```python
from build123d import *

# Parameters (mm, degrees)
F1_DEPTH  = 75
F2_W      = 55
F2_H      = 95
F3_DEPTH  = 3.001
F5_DEPTH  = 55
F7_DEPTH  = 3
F9_DEPTH  = 3
F10_R     = 2
F12_DEPTH = 3
F13_W     = 4
F13_H     = 3.0462798357
F14_DEPTH = 1


with BuildPart() as f1:
    # F0 (on Front) → F1 (new body)
    with BuildSketch(Plane.XZ):
        with BuildLine():
            Line((-3, 0), (0, 0))
            Line((0, 0), (0, 146.328642619))
            ThreePointArc((0, 146.328642619), (1.7690799336, 150.0361338491), (5.6451438845, 151.3967452123))
            Line((5.6451438845, 151.3967452123), (79.5057253604, 138.3731318873))
            Line((79.5057253604, 138.3731318873), (79.5057253604, 141.4194117229))
            Line((79.5057253604, 141.4194117229), (6.010801042, 154.3785498254))
            ThreePointArc((6.010801042, 154.3785498254), (-0.193413929, 152.3056303595), (-3, 146.396962731))
            Line((-3, 146.396962731), (-3, 146.1928579517))
            Line((-3, 146.1928579517), (-3, 0))
        make_face()
    extrude(amount=-F1_DEPTH)

    # F2 (on face) → F3 (cut, through all)
    with BuildSketch(Plane.YZ):
        with Locations((37.5, 47.5)):
            Rectangle(F2_W, F2_H)
    extrude(amount=-F3_DEPTH, mode=Mode.SUBTRACT)

    # F4 (on face) → F5 (join)
    with BuildSketch(Plane.XZ.offset(-65)):
        Polygon((0, 95), (-3, 95), (32.2094485164, 0), (47.2094485164, 0), (47.2094485164, 3), (34.2969885133, 3), align=None)
    extrude(amount=F5_DEPTH)

    # F6 (on face) → F7 (cut)
    with BuildSketch(Plane(origin=(0, 0, 0), x_dir=(1, 0, 0), z_dir=(0, 0, -1))):
        with BuildLine():
            ThreePointArc((42.2094485164, -37.5), (41.4772154693, -35.732233047), (39.7094485164, -35))
            Line((39.7094485164, -35), (39.7094485164, -40))
            ThreePointArc((39.7094485164, -40), (41.4772154693, -39.267766953), (42.2094485164, -37.5))
        make_face()
        with BuildLine():
            Line((39.7094485164, -40), (39.7094485164, -35))
            ThreePointArc((39.7094485164, -35), (37.2094485164, -37.5), (39.7094485164, -40))
        make_face()
    extrude(amount=-F7_DEPTH, mode=Mode.SUBTRACT)

    # F8 (on face) → F9 (cut, through all)
    with BuildSketch(Plane.YZ):
        with BuildLine():
            Line((7, 6), (7, 12))
            ThreePointArc((7, 12), (5, 14), (3, 12))
            Line((3, 12), (3, 6))
            ThreePointArc((3, 6), (5, 4), (7, 6))
        make_face()
        with BuildLine():
            ThreePointArc((72, 12), (70, 14), (68, 12))
            Line((68, 12), (68, 6))
            ThreePointArc((68, 6), (70, 4), (72, 6))
            Line((72, 6), (72, 12))
        make_face()
    extrude(amount=-F9_DEPTH, mode=Mode.SUBTRACT)

    # F10
    f10_edges = [f1.edges().sort_by_distance(p)[0] for p in [
        (32.209449, 37.5, 0),
        (34.296989, 37.5, 3),
    ]]
    fillet(f10_edges, radius=F10_R)

    # F11 (on face) → F12 (cut, through all)
    with BuildSketch(Plane(origin=(26.5815346978, 0, 150.7513744689), x_dir=(0.984807753, 0, -0.1736481777), z_dir=(0.1736481777, 0, 0.984807753))):
        with BuildLine():
            Line((53.7406316114, 23.6), (33.7406316114, 23.6))
            ThreePointArc((33.7406316114, 23.6), (31.7406316114, 21.6), (33.7406316114, 19.6))
            Line((33.7406316114, 19.6), (53.7406316114, 19.6))
            Line((53.7406316114, 19.6), (53.7406316114, 23.6))
        make_face()
        with BuildLine():
            Line((13.7406316114, 51.4), (33.7406316114, 51.4))
            Line((33.7406316114, 51.4), (53.7406316114, 51.4))
            Line((53.7406316114, 51.4), (53.7406316114, 55.4))
            Line((53.7406316114, 55.4), (13.7406316114, 55.4))
            ThreePointArc((13.7406316114, 55.4), (11.7406316114, 53.4), (13.7406316114, 51.4))
        make_face()
    extrude(amount=-F12_DEPTH, mode=Mode.SUBTRACT)

    # F13 (on face) → F14 (cut)
    with BuildSketch(Plane.YZ.offset(79.5057253604)):
        with Locations((21.6, 139.8962718051)):
            Rectangle(F13_W, F13_H)
        with Locations((53.4, 139.8962718051)):
            Rectangle(F13_W, F13_H)
    extrude(amount=-F14_DEPTH, mode=Mode.SUBTRACT)


solid = f1.part
```
Model file for the job. Use its own axes, mm. A direction names the side the tool comes from. Round coordinates to 2 decimals unless told otherwise and drop trailing zeros. Write each loop counter-clockwise with the first axis right and the second up, starting at its lowest first coordinate (ties: lowest second). Pieces come first, ordered by that corner, then holes. Notation, with made-up numbers: (-27.5, 82) - (-13.5, 82) arc R15 cw to (-13.5, 109) - close; hole circle Ø2 at (-29.75, -9). An arc over 180 degrees is marked (long way). One line per item, written item: value.
(1) Wall check: probe 1 along X at (y, z) = (48, 87) (3 decimals); probe 2 along X at (y, z) = (3, 37); probe 3 along Z at (x, y) = (67, 40.5). Give the ranges that are in metal, low to high.
Values follow:
probe 1: x = -0.035 to 2.982
probe 2: x = -3 to 0
probe 3: z = 140.58 to 143.62
(2) Two-plate mould, pull along Y, no slides. Class faces 5 (the flat face through (-1, 72, 9)), 6 (the flat face through (-2, 75, 100)), 7 (the flat face through (79.506, 37, 140)): pulls with the +Y half, pulls with the -Y half, needs draft (parallel to the pull), parting line crosses it, or undercut.
Values follow:
face 5: undercut
face 6: pulls with the +Y half
face 7: needs draft
(3) Drop flat-ended pins along their axis: P1, Ø6, axis at x = 43, y = 28.5, coming from the +Z side; P2, Ø8, axis at y = 49, z = 73.5, coming from the +X side; P3, Ø14, axis at x = 15, z = 30.5, coming from the +Y side. Give the stop position or say it passes through.
Values follow:
P1: stops at z = 148.39
P2: stops at x = 9.51
P3: stops at y = 65
(4) Cut at A-A, the plane y = 5. Give the cut face in (x, z).
Values follow:
outline: (-3, 0) - (0, 0) - (0, 4) - (-3, 4) - close; (-3, 14) - (0, 14) - (0, 146.33) arc R5.35 cw to (5.65, 151.4) - (79.51, 138.37) - (79.51, 141.42) - (6.01, 154.38) arc R8.35 ccw to (-3, 146.4) - close
(5) Cut at D-D, the plane x = 27.5. Give the cut face in (y, z), plus the area to 3 significant figures.
Values follow:
outline: (0, 147.54) - (75, 147.54) - (75, 150.59) - (0, 150.59) - close; (10, 12.71) - (65, 12.71) - (65, 21.23) - (10, 21.23) - close
area: 697 mm²
(6) 3-axis set-ups, long thin cutter, end or side, ignore diameter. For faces 1 (the flat face through (47.209, 38, 1)), 2 (the flat face through (17.14, 37.89, 49.02)), 3 (the flat face through (60, 51.4, 143)), 4 (the cylindrical face through (-1, 70, 4)): which of +Z, -Z, +X, -X, +Y, -Y reach the whole face in a straight line?
Values follow:
face 1: -Z, +X, +Y, -Y
face 2: +X, +Y, -Y
face 3: +Z, +X
face 4: +X, -X
(7) Cut at C-C, the plane x = 65. Give the cut face in (y, z), plus the area to 3 significant figures.
Values follow:
outline: (0, 140.93) - (19.6, 140.93) - (19.6, 143.98) - (0, 143.98) - close; (23.6, 140.93) - (51.4, 140.93) - (51.4, 143.98) - (23.6, 143.98) - close; (55.4, 140.93) - (75, 140.93) - (75, 143.98) - (55.4, 143.98) - close
area: 204 mm²
(8) Cut at B-B, the plane z = 52. Give the cut face in (x, y), plus the area to 3 significant figures.
Values follow:
outline: (-3, 0) - (0, 0) - (0, 10) - (-3, 10) - close; (-3, 65) - (0, 65) - (0, 75) - (-3, 75) - close; (12.94, 10) - (16.03, 10) - (16.03, 65) - (12.94, 65) - close
area: 230 mm²
